For this review, use the dimensioned drawing (mm, ordinates from the lowest corner) and the shaded views. Coordinates: 2 decimals unless noted, no trailing zeros. Loops run counter-clockwise (first coordinate to the right, second up) from the corner with the lowest first, then second, coordinate; pieces in that order, holes last.
1. Take a section at B-B, the plane y = 3.25. State the section outline as (x, z) points.
2. Clearance check with flat-ended pins moving along their axes: P1, Ø6, axis at x = 6, z = 6.5, coming from the +Y side; P2, Ø1, axis at x = 5.5, y = 6, coming from the -Z side; P3, Ø2, axis at x = 1.5, y = 8, coming from the -Z side. State where each tip first meets the part, or that it passes through.
3. To check wall thickness, follow probe 1 along Y at (x, z) = (5.5, 2); probe 2 along Y at (x, z) = (8.75, 6.25); probe 3 along Z at (x, y) = (6.25, 4). State the ranges of each line that lie inside material, in increasing order.
4. Take a section at C-C, the plane z = 1. State the section outline as (x, y) points.
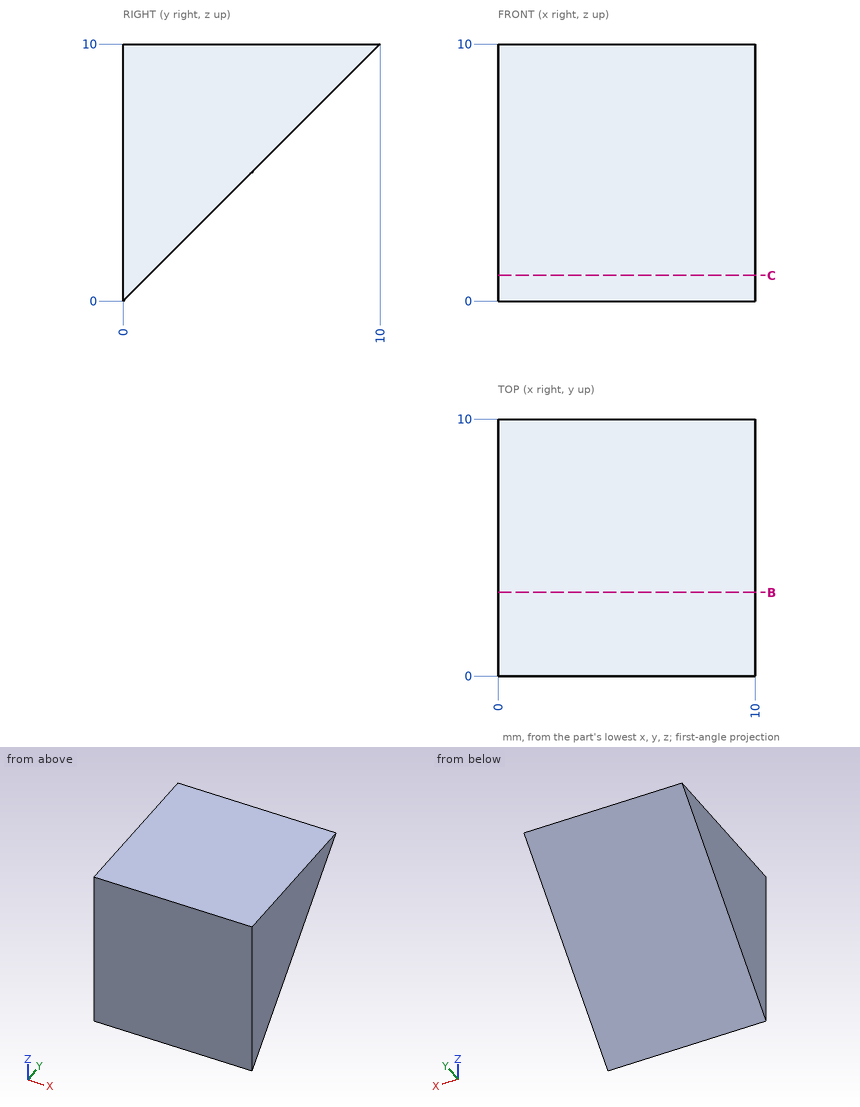
Results list:
1. outline: (0, 3.25) - (10, 3.25) - (10, 10) - (0, 10) - close
2. P1: stops at y = 9.5
2. P2: stops at z = 5.5
2. P3: stops at z = 7
3. probe 1: y = 0 to 2
3. probe 2: y = 0 to 6.25
3. probe 3: z = 4 to 10
4. outline: (0, 0) - (10, 0) - (10, 1) - (0, 1) - close
